Work out the finished part from the listing and answer in its coordinate system (mm). Face numbers are marked on the shaded views. A direction names the side the tool comes from. Coordinates: 2 decimals unless noted, no trailing zeros. Write each loop counter-clockwise with the first axis right and the second up, starting at its lowest first coordinate (ties: lowest second). Pieces come first, ordered by that corner, then holes. Notation, with made-up numbers: (64.5, -30) - (76.5, -30) arc R11 ccw to (76.5, -12) - close; hole circle Ø3 at (84.25, 45.5). An arc over 180 degrees is marked (long way). Use one line per item in the form item = value. Start each with the question number.
Item 1: Consider probe 1 along Z at (x, y) = (53.5, 51.5); probe 2 along Z at (x, y) = (10.5, 67); probe 3 along Y at (x, z) = (19.5, 10.75). Determine where each line is inside the solid, lowest interval first.
Item 2: For the marked faces 1, 2, 3 and 4, determine the directions among +Z, -Z, +X, -X, +Y, -Y from which every point of the face is accessible in a straight line to the end or side of a thin tool.
Item 3: A cutting plane is placed at B-B (y = 68). Write down the section's boundary in (x, z), then the cut area to 3 significant figures.
Item 4: A cutting plane is placed at A-A (x = 8.5). Write down the section's boundary in (y, z), then the cut area to 3 significant figures.
Item 5: Given pin 1 (1 mm diameter, centred on y = 51, z = 8.5, fed in from +X); pin 2 (4 mm diameter, centred on y = 47.5, z = 11, fed in from +X); pin 3 (4 mm diameter, centred on y = 7, z = 15.5, fed in from -X), each flat-ended and moving along its own axis, determine where each tip first touches the part or whether it passes through.
Item 6: A cutting plane is placed at C-C (z = 10.75). Write down the section's boundary in (x, y).
from build123d import *

# Parameters (mm, degrees)
F0_W     = 76.2
F0_H     = 76.2
F1_DEPTH = 5.842
F2_R     = 38.1
F3_DEPTH = 5.842
F5_DEPTH = 5.842


with BuildPart() as f1:
    # F0 (on Top) → F1 (new body)
    with BuildSketch(Plane.XY):
        with Locations((32.087865, 34.309075)):
            Rectangle(F0_W, F0_H)
    extrude(amount=F1_DEPTH)

    # F2 (on face) → F3 (join)
    with BuildSketch(Plane.XY.offset(5.842)):
        with Locations((32.087865, 34.309075)):
            Circle(F2_R)
    extrude(amount=F3_DEPTH)

    # F4 (on face) → F5 (join)
    with BuildSketch(Plane.XY.offset(11.684)):
        Polygon((70.187865, 34.309075), (32.087865, 72.409075), (-6.012135, 34.309075), (32.087865, -3.790925), align=None)
    extrude(amount=F5_DEPTH)


solid = f1.part
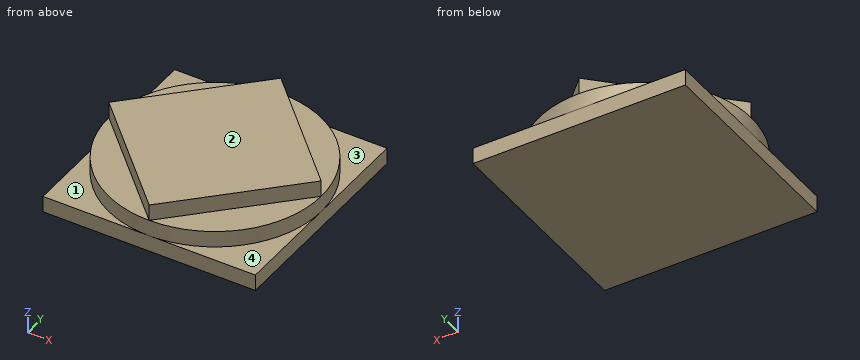
Answer:
q1.probe_1 = 0 to 11.68
q1.probe_2 = 0 to 5.84
q1.probe_3 = -1.65 to 70.27
q2.face_1 = +Z, -X, -Y
q2.face_2 = +Z, +X, -X, +Y, -Y
q2.face_3 = +Z, +X, +Y
q2.face_4 = +Z, +X, -Y
q3.outline = (-6.01, 0) - (70.19, 0) - (70.19, 5.84) - (49.88, 5.84) - (49.88, 11.68) - (36.5, 11.68) - (36.5, 17.53) - (27.68, 17.53) - (27.68, 11.68) - (14.3, 11.68) - (14.3, 5.84) - (-6.01, 5.84) - close
q3.area = 705 mm²
q4.outline = (-3.79, 0) - (72.41, 0) - (72.41, 5.84) - (64.23, 5.84) - (64.23, 11.68) - (48.82, 11.68) - (48.82, 17.53) - (19.8, 17.53) - (19.8, 11.68) - (4.39, 11.68) - (4.39, 5.84) - (-3.79, 5.84) - close
q4.area = 964 mm²
q5.pin_1 = 66.58
q5.pin_2 = 68.51
q5.pin_3 = 19.3
q6.outline = circle Ø76.2 at (32.09, 34.31)
